For this review, take the finished solid that the model builds, in its own axes (mm). A direction names the side the tool comes from. Give positions to 0.01 mm unless a question says otherwise; leave off trailing zeros. Loops run counter-clockwise (first coordinate to the right, second up) from the corner with the lowest first, then second, coordinate; pieces in that order, holes last.
```python
from build123d import *

# Parameters (mm, degrees)
F0_W     = 600
F0_H     = 400
F1_DEPTH = 20
F2_R     = 6.25
F3_DEPTH = 25
F4_R     = 9.5
F5_DEPTH = 13


with BuildPart() as f1:
    # F0 (on Top) → F1 (new body)
    with BuildSketch(Plane.XY):
        Rectangle(F0_W, F0_H)
    extrude(amount=F1_DEPTH)

    # F2 (on face) → F3 (cut)
    with BuildSketch(Plane.XY.offset(20)):
        with Locations((-250, 125)):
            Circle(F2_R)
        with Locations((-250, -125)):
            Circle(F2_R)
        with Locations((250, 125)):
            Circle(F2_R)
        with Locations((250, -125)):
            Circle(F2_R)
        Circle(F2_R)
    extrude(amount=-F3_DEPTH, mode=Mode.SUBTRACT)

    # F4 (on face) → F5 (cut)
    with BuildSketch(Plane.XY.offset(20)):
        with Locations((250, 125)):
            Circle(F4_R)
        with Locations((250, -125)):
            Circle(F4_R)
        Circle(F4_R)
        with Locations((-250, 125)):
            Circle(F4_R)
        with Locations((-250, -125)):
            Circle(F4_R)
    extrude(amount=-F5_DEPTH, mode=Mode.SUBTRACT)


solid = f1.part
```
Q1. Mouldability with a two-part tool opening along Y and no side actions: class faces 3 (the flat face through (-300, -3, 10)), 4 (the flat face through (-4, -200, 10)), 5 (the cylindrical face through (-245.62, 116.57, 13.59)), 6 (the flat face through (252, 118.8, 7)) as +Y half, -Y half, draft (parallel to the pull), parting line (faces both ways), or undercut.
Answers:
face 3: draft
face 4: -Y half
face 5: undercut
face 6: undercut
Q2. Consider section B-B on x = 0. Give the boundary of the cut face in (y, z), plus the area to 3 significant figures.
Answers:
outline: (-200, 0) - (-6.25, 0) - (-6.25, 7) - (-9.5, 7) - (-9.5, 20) - (-200, 20) - close; (6.25, 0) - (200, 0) - (200, 20) - (9.5, 20) - (9.5, 7) - (6.25, 7) - close
area: 7,670 mm2
Q3. Machinability: for faces 1 (the flat face through (6.2, -2, 7)), 2 (the flat face through (-4, 47, 0)), which of the approach directions +Z, -Z, +X, -X, +Y, -Y give a long, thin tool a straight path to every point of the face, cutting with its end or side? Answer none if there is none.
Answers:
face 1: +Z
face 2: -Z, +X, -X, +Y, -Y
Q4. Consider section C-C on y = -125. Give the boundary of the cut face in (x, z), plus the area to 3 significant figures.
Answers:
outline: (-300, 0) - (-256.25, 0) - (-256.25, 7) - (-259.5, 7) - (-259.5, 20) - (-300, 20) - close; (-243.75, 0) - (243.75, 0) - (243.75, 7) - (240.5, 7) - (240.5, 20) - (-240.5, 20) - (-240.5, 7) - (-243.75, 7) - close; (256.25, 0) - (300, 0) - (300, 20) - (259.5, 20) - (259.5, 7) - (256.25, 7) - close
area: 11,300 mm2
Q5. Consider section D-D on x = 250. Give the boundary of the cut face in (y, z), plus the area to 3 significant figures.
Answers:
outline: (-200, 0) - (-131.25, 0) - (-131.25, 7) - (-134.5, 7) - (-134.5, 20) - (-200, 20) - close; (-118.75, 0) - (118.75, 0) - (118.75, 7) - (115.5, 7) - (115.5, 20) - (-115.5, 20) - (-115.5, 7) - (-118.75, 7) - close; (131.25, 0) - (200, 0) - (200, 20) - (134.5, 20) - (134.5, 7) - (131.25, 7) - close
area: 7,330 mm2
Q6. For pin 1 Ø9.5 at (x, y) = (-0.5, 3) entering from +Z; pin 2 Ø11.5 at (x, y) = (0, 0) entering from +Z, all flat-tipped, find the tip position at first contact; note any pin that passes through.
Answers:
pin 1: stops at z = 7
pin 2: passes through
Q7. Consider section A-A on y = 0. Give the boundary of the cut face in (x, z), plus the area to 3 significant figures.
Answers:
outline: (-300, 0) - (-6.25, 0) - (-6.25, 7) - (-9.5, 7) - (-9.5, 20) - (-300, 20) - close; (6.25, 0) - (300, 0) - (300, 20) - (9.5, 20) - (9.5, 7) - (6.25, 7) - close
area: 11,700 mm2
Q8. For probe 1 along Y at (x, z) = (250, 14); probe 2 along X at (y, z) = (-120.5, 18.75), list the stretches that pass through material, from the lowest coordinate up.
Answers:
probe 1: y = -200 to -134.5, -115.5 to 115.5, 134.5 to 200
probe 2: x = -300 to -258.37, -241.63 to 241.63, 258.37 to 300
